CAD build for the part. Positions are in the model's coordinates, mm. Face numbers are marked on the shaded views. Coordinates: 2 decimals unless noted, no trailing zeros. Order: outer loops, then holes, each group sorted by start corner. A loop starts at its lowest first (then second) coordinate and runs counter-clockwise, first axis right, second up. Notation, with made-up numbers: M -17.5,37.25 L 1.5,37.25 A28 ccw 1.5,68.25 Z; hole C 15,59.5 d4. An arc over 180 degrees is marked long. Write item = value, one per line.
from build123d import *


with BuildPart() as part:
    # Esquisse2 → Base-Révolution (revolve)
    with BuildSketch(Plane(origin=(0, 0, 0), x_dir=(1, 0, 0), z_dir=(0, 1, 0)), mode=Mode.PRIVATE) as base_r_volution_sk:
        Polygon((0, -25), (0, -27), (-10, -27), (-10, -28), (0, -28), (5, -26), (5, -25), align=None)
    revolve(base_r_volution_sk.sketch.rotate(Axis((37.900503033, 0, 0), (-1, 0, 0)), 180), axis=Axis((37.900503033, 0, 0), (-1, 0, 0)))


solid = part.part
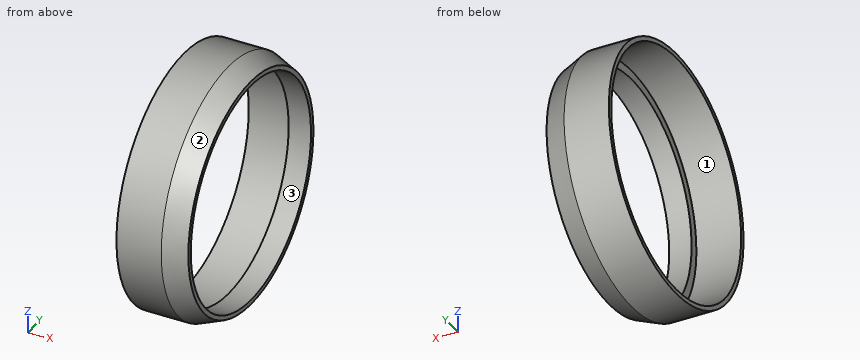
(1) Pull direction Z, two halves, no side cores. Call the marked faces 1, 2 and 3: +Z half, -Z half, draft (parallel to the pull), parting line (faces both ways), or undercut.
Evaluation:
face_1 = undercut
face_2 = parting line
face_3 = undercut
(2) Slice it at A-A, the plane z = 0. Write the cut outline in (x, y), then the cut area to 3 significant figures.
Evaluation:
outline = M -10,-28 L 0,-28 L 5,-26 L 5,-25 L 0,-25 L 0,-27 L -10,-27 Z; M -10,27 L 0,27 L 0,25 L 5,25 L 5,26 L 0,28 L -10,28 Z
area = 40.0 mm²
(3) Pin check, flat tips, straight feed: pin 1 Ø6 at (x, y) = (2, -21.5) entering from +Z; pin 2 Ø1 at (x, z) = (-2.5, 10.5) entering from -Y; pin 3 Ø5 at (x, z) = (3.5, 13.5) entering from -Y; pin 4 Ø12 at (y, z) = (11, 9) entering from -X. Stop position of each tip, or through.
Evaluation:
pin_1 = 20.39
pin_2 = -26.15
pin_3 = -24.66
pin_4 = through
(4) Slice it at B-B, the plane x = -8. Write the cut outline in (y, z).
Evaluation:
outline = C 0,0 d56; hole C 0,0 d54
(5) Wall check: line 1 (Y direction, x = -5, z = 0); line 2 (Y direction, x = -5.75, z = -11.5); line 3 (Z direction, x = -7, y = -20.5). Give the ranges that are in metal, low to high. Write a range as from..to.
Evaluation:
line_1 = -28..-27, 27..28
line_2 = -25.53..-24.43, 24.43..25.53
line_3 = -19.07..-17.57, 17.57..19.07
